Here's how the part is built. I have some questions about the finished solid (model axes, mm). A direction names the side the tool comes from. Give positions to 0.01 mm unless a question says otherwise; leave off trailing zeros. Loops run counter-clockwise (first coordinate to the right, second up) from the corner with the lowest first, then second, coordinate; pieces in that order, holes last. Notation, with made-up numbers: (-31, -3.5) -> (-15, -3.5) arc R22 cw to (-15, 23.5) -> close; hole circle Ø3 at (-9, 46). An arc over 180 degrees is marked (long way). Answer in a Markdown table with one row per item. Add a question column.
Item 1: We'd pull the mould along X, two halves only. Please class faces 5 (the face through (17.5, -1, 15)), 6 (the face through (1, 10, 10)), 7 (the face through (27.5, -1, -15)), 8 (the face through (45.252, 26.014, 4.901)): released by +X, released by -X, zero draft, split by the parting line, or undercut.
Item 2: Which directions (+Z, -Z, +X, -X, +Y, -Y) give clear straight access to the entire face, cutting with the end or side of a thin tool? Please do faces 1 (the face through (43, 13, 0)), 2 (the face through (0, 11, 0)), 3 (the face through (17.5, -1, -15)), 4 (the face through (45, 11, 0)).
Item 3: If we section it at A-A (z = -15): Write out the boundary of the cut face in (x, y).
Item 4: If we section it at D-D (z = 5): Write out the boundary of the cut face in (x, y).
Item 5: If we section it at C-C (y = 16): Write out the boundary of the cut face in (x, z).
Item 6: If I drill on line 1 (Z direction, x = 47.5, y = 26.55); line 2 (X direction, y = 26.05, z = 5); line 3 (X direction, y = 18.5, z = 4), over which ranges is the centre line in solid material (lowest first)?
Item 7: If we section it at B-B (x = -2.5): Write out the boundary of the cut face in (y, z), then the cut area to 3 significant figures.
Item 8: For P1, Ø8, axis at x = 50, z = -2.5, coming from the -Y side; P2, Ø7.5, axis at x = -0.5, y = 15, coming from the +Z side; P3, Ø1.6, axis at y = -1.5, z = 16.5, coming from the -X side, each with a flat end and sliding along its axis, tell me the tip position at first contact or that it passes through.
Autodesk Inventor part; units mm, degrees
ref_plane "YZ Plane" through (0, 0, 0) normal (1, 0, 0) x (0, 1, 0)
ref_plane "XZ Plane" through (0, 0, 0) normal (0, 1, 0) x (-1, 0, 0)
ref_plane "XY Plane" through (0, 0, 0) normal (0, 0, 1) x (1, 0, 0)
sketch "Sketch1" plane through (0, 0, 0) normal (0, 0, 1) x (1, 0, 0)
  line L0 (2, 0) -> (43, 0)
  line L1 (45, 0) -> (45, -2)
  line L2 (45, -2) -> (0, -2)
  line L3 (0, -2) -> (0, 0)
  line L4 (45, 0) -> (45, 25)
  line L5 (52.3, 27) -> (52.3, 25)
  line L6 (52.3, 25) -> (45, 25)
  line L7 (22.5, -2) -> (22.5, 38) construction
  line L8 (0, 0) -> (0, 25)
  line L9 (-7.3, 27) -> (-7.3, 25)
  line L10 (-7.3, 25) -> (0, 25)
  line L11 (2, 0) -> (2, 27)
  line L12 (43, 0) -> (43, 27)
  line L13 (43, 27) -> (52.3, 27)
  line L14 (-7.3, 27) -> (2, 27)
  line L15 (17.5, -2) -> (17.5, 0)
  line L16 (27.5, -2) -> (27.5, 0)
  point P0 (27.5, -2)
  point P1 (17.5, -2)
  dimension "d0" = 45
  dimension "d4" = 2
  dimension "d5" = 40
  dimension "d8" = 2
  dimension "d9" = 27
  dimension "d11" = 9.3
  dimension "d20" = 2
  dimension "d29" = 5
  dimension "d30" = 10
extrude "Extrusion1" add sketch "Sketch1" along normal mid plane 20 contours L0 L15 L2 L3 L8 L10 L9 L14 L11 | L0 L12 L13 L5 L6 L4 L1 L2 L16
sketch "Sketch3" plane through (-7.3, 27, -10) normal (0, 1, 0) x (1, 0, 0)
  circle A0 centre (4.8, -5) radius 2.25
  line L0 (9.3, 0) -> (9.3, -20)
  line L1 (0, 0) -> (9.3, 0)
  circle A1 centre (4.8, -15) radius 2.25
  line L2 (7.3, -20) -> (52.3, -20) construction
  line L3 (29.8, -20) -> (29.8, 0) construction
  circle A2 centre (54.8, -5) radius 2.25
  circle A3 centre (54.8, -15) radius 2.25
  dimension "d21" = 4.5
  dimension "d22" = 4.5
  dimension "d23" = 5
  dimension "d24" = 4.5
  dimension "d25" = 10
  dimension "d26" = 4.5
extrude "Extrusion2" cut sketch "Sketch3" against normal through all
extrude "Extrusion3" add sketch "Sketch1" along normal mid plane 40 contours L0 L16 L2 L15
sketch "Sketch4" plane through (2, 0, 10) normal (0, 1, 0) x (1, 0, 0)
  circle A0 centre (20.5, -5) radius 2.5
  circle A1 centre (20.5, 25) radius 2.5
  line L0 (15.5, 30) -> (25.5, 30)
  line L1 (25.5, 20) -> (25.5, 30)
  line L2 (25.5, -10) -> (25.5, 0)
  line L3 (25.5, -10) -> (15.5, -10)
  point P0 (-2, 10)
  dimension "d33" = 5
  dimension "d34" = 5
  dimension "d35" = 5
  dimension "d36" = 5
  dimension "d37" = 5
extrude "Extrusion4" cut sketch "Sketch4" against normal blind 5
thread "Thread1"
thread "Thread2"
thread "Thread3"
thread "Thread4"
thread "Thread5"
thread "Thread6"
equation "\"d11\" = d10"
equation "\"d26\" = d22"
equation "\"d36\" = d34"
equation "\"d37\" = d33"
equation "\"d38\" = d37"
properties part number "Servo Mount"
Recorded:
| question | item | result |
|---|---|---|
| 1 | face 5 | released by -X |
| 1 | face 6 | zero draft |
| 1 | face 7 | released by +X |
| 1 | face 8 | undercut |
| 2 | face 1 | +Z, -Z, +Y |
| 2 | face 2 | +Z, -Z, -X, -Y |
| 2 | face 3 | -Z, -X, +Y, -Y |
| 2 | face 4 | +Z, -Z, +X, -Y |
| 3 | outline | (17.5, -2) -> (20, -2) -> (20, 0) -> (17.5, 0) -> close; (25, -2) -> (27.5, -2) -> (27.5, 0) -> (25, 0) -> close |
| 4 | outline | (-7.3, 25) -> (-4.75, 25) -> (-4.75, 27) -> (-7.3, 27) -> close; (-0.25, 25) -> (0, 25) -> (0, -2) -> (45, -2) -> (45, 25) -> (45.25, 25) -> (45.25, 27) -> (43, 27) -> (43, 0) -> (2, 0) -> (2, 27) -> (-0.25, 27) -> close; (49.75, 25) -> (52.3, 25) -> (52.3, 27) -> (49.75, 27) -> close |
| 5 | outline | (0, -10) -> (2, -10) -> (2, 10) -> (0, 10) -> close; (43, -10) -> (45, -10) -> (45, 10) -> (43, 10) -> close |
| 6 | line 1 | z = -10 to -7.25, -2.75 to 2.75, 7.25 to 10 |
| 6 | line 2 | x = -7.3 to -4.75, -0.25 to 2, 43 to 45.25, 49.75 to 52.3 |
| 6 | line 3 | x = 0 to 2, 43 to 45 |
| 7 | outline | (25, -10) -> (27, -10) -> (27, -7.25) -> (25, -7.25) -> close; (25, -2.75) -> (27, -2.75) -> (27, 2.75) -> (25, 2.75) -> close; (25, 7.25) -> (27, 7.25) -> (27, 10) -> (25, 10) -> close |
| 7 | area | 22.0 mm^2 |
| 8 | P1 | stops at y = 25 |
| 8 | P2 | stops at z = 10 |
| 8 | P3 | stops at x = 17.5 |
